Design review of the part built by this model. Coordinates are the model's own, in mm. Face numbers are marked on the shaded views. Round coordinates to 2 decimals unless told otherwise and drop trailing zeros. Loops run counter-clockwise (first coordinate to the right, second up) from the corner with the lowest first, then second, coordinate; pieces in that order, holes last. Notation, with made-up numbers: M 79,0 L 89,0 A24 cw 89,18 Z; hole C -31,6.25 d7. An arc over 180 degrees is marked long. One line per item, written item: value. Start each with the question number.
Item 1: We need section B-B (z = 51.5). Write out the cut boundary in (x, y).
Item 2: We need section C-C (y = 23.5). Write out the cut boundary in (x, z).
Item 3: For line 1 along Z through (x, y) = (0, 35.5); line 2 along X through (y, z) = (31, 140); line 3 along X through (y, z) = (42, 140), list the stretches that pass through material, from the lowest coordinate up.
Item 4: Clearance check with flat-ended pins moving along their axes: pin 1 (4.5 mm diameter, centred on x = 0.5, z = 30.5, fed in from -Y); pin 2 (3 mm diameter, centred on x = -0.5, z = 140.5, fed in from +Y); pin 3 (8 mm diameter, centred on y = 40.5, z = 32.5, fed in from -X); pin 4 (8 mm diameter, centred on x = 54, z = 77.5, fed in from -Y). State where each tip first meets the part, or that it passes through.
Item 5: Mouldability with a two-part tool opening along Y and no side actions: class the marked faces 1, 2 and 3 as released by +Y, released by -Y, zero draft, split by the parting line, or undercut.
Item 6: We need section A-A (x = 0). Write out the cut boundary in (y, z), then the cut area to 3 significant figures.
Item 7: We need section D-D (y = -2.5). Write out the cut boundary in (x, z), then the cut area to 3 significant figures.
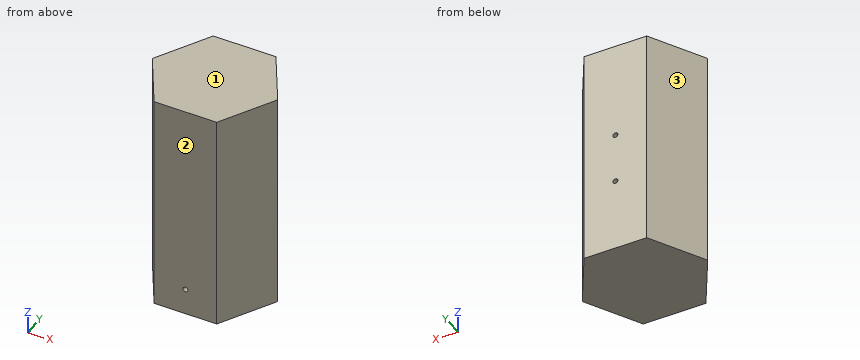
from build123d import *

# Parameters (mm, degrees)
F1_DEPTH = 250
F3_D     = 5.5
F3_DEPTH = 61.0402304845
F4_D     = 5.5
F4_DEPTH = 61.0402304845


with BuildPart() as f1:
    # F0 (on Top) → F1 (new body)
    with BuildSketch(Plane.XY):
        Polygon((35.2410161514, -61.0392304845), (70.4820323028, 0), (35.2410161514, 61.0392304845), (-35.2410161514, 61.0392304845), (-70.4820323028, 0), (-35.2410161514, -61.0392304845), align=None)
    extrude(amount=F1_DEPTH)

    # F3 (through all, one way)
    with BuildSketch(Plane.XZ):
        with Locations((0, 140), (0, 83)):
            Circle(F3_D / 2)
    extrude(amount=-F3_DEPTH, mode=Mode.SUBTRACT)

    # F4 (through all, one way)
    with BuildSketch(Plane(origin=(0, 0, 0), x_dir=(1, 0, 0), z_dir=(0, 1, 0))):
        with Locations((0, -30)):
            Circle(F4_D / 2)
    extrude(amount=-F4_DEPTH, mode=Mode.SUBTRACT)


solid = f1.part
A:
1. outline: M -70.48,0 L -35.24,-61.04 L 35.24,-61.04 L 70.48,0 L 35.24,61.04 L -35.24,61.04 Z
2. outline: M -56.91,0 L 56.91,0 L 56.91,250 L -56.91,250 Z; hole C 0,83 d5.5; hole C 0,140 d5.5
3. line 1: 0 to 80.25, 85.75 to 137.25, 142.75 to 250
3. line 2: -52.58 to -2.75, 2.75 to 52.58
3. line 3: -46.23 to -2.75, 2.75 to 46.23
4. pin 1: y = -61.04
4. pin 2: y = 0
4. pin 3: x = -49.41
4. pin 4: y = -35.48
5. face 1: zero draft
5. face 2: released by -Y
5. face 3: released by +Y
6. outline: M -61.04,0 L 61.04,0 L 61.04,80.25 L 0,80.25 L 0,85.75 L 61.04,85.75 L 61.04,137.25 L 0,137.25 L 0,142.75 L 61.04,142.75 L 61.04,250 L -61.04,250 L -61.04,32.75 L 0,32.75 L 0,27.25 L -61.04,27.25 Z
6. area: 29,500 mm2
7. outline: M -69.04,0 L 69.04,0 L 69.04,250 L -69.04,250 Z; hole C 0,30 d5.5
7. area: 34,500 mm2
